from build123d import *

# Parameters (mm, degrees)
SKETCH1_W           = 121
SKETCH1_H           = 66
BOSS_EXTRUDE1_DEPTH = 3.8
SKETCH2_W           = 109
SKETCH2_H           = 58
CUT_EXTRUDE1_DEPTH  = 4.8
FILLET1_R           = 5
SKETCH3_W           = 20
SKETCH3_H           = 58
BOSS_EXTRUDE2_DEPTH = 3.8
FILLET2_R           = 3
SKETCH4_R           = 1
CUT_EXTRUDE2_DEPTH  = 4.8
BOSS_EXTRUDE3_DEPTH = 3.8
FILLET3_R           = 3
SKETCH6_W           = 3.8
SKETCH6_H           = 10
SKETCH6_W_2         = 10
SKETCH6_H_2         = 3.8
CUT_EXTRUDE3_DEPTH  = 4.8


with BuildPart() as part:
    # Sketch1 → Boss-Extrude1 (new body)
    with BuildSketch(Plane(origin=(0, 0, 0), x_dir=(1, 0, 0), z_dir=(0, 1, 0))):
        with Locations((60.5, -33)):
            Rectangle(SKETCH1_W, SKETCH1_H)
    extrude(amount=BOSS_EXTRUDE1_DEPTH)

    # Sketch2 → Cut-Extrude1 (cut, through all)
    with BuildSketch(Plane(origin=(0, 3.8, 0), x_dir=(1, 0, 0), z_dir=(0, 1, 0))):
        with Locations((60.5, -33)):
            Rectangle(SKETCH2_W, SKETCH2_H)
    extrude(amount=-CUT_EXTRUDE1_DEPTH, mode=Mode.SUBTRACT)

    # Fillet1
    fillet1_edges = [part.edges().sort_by_distance(p)[0] for p in [
        (115, 1.9, 4),
        (115, 1.9, 62),
        (6, 1.9, 62),
        (6, 1.9, 4),
    ]]
    fillet(fillet1_edges, radius=FILLET1_R)

    # Sketch3 → Boss-Extrude2 (add, through all)
    with BuildSketch(Plane(origin=(0, 3.8, 0), x_dir=(1, 0, 0), z_dir=(0, 1, 0))):
        with Locations((60.5, -33)):
            Rectangle(SKETCH3_W, SKETCH3_H)
    extrude(amount=-BOSS_EXTRUDE2_DEPTH)

    # Fillet2
    fillet2_edges = [part.edges().sort_by_distance(p)[0] for p in [
        (70.5, 1.9, 4),
        (70.5, 1.9, 62),
        (50.5, 1.9, 62),
        (50.5, 1.9, 4),
    ]]
    fillet(fillet2_edges, radius=FILLET2_R)

    # Sketch4 → Cut-Extrude2 (cut, through all)
    with BuildSketch(Plane(origin=(0, 3.8, 0), x_dir=(1, 0, 0), z_dir=(0, 1, 0))):
        with Locations((116.5, -61.5)):
            Circle(SKETCH4_R)
        with Locations((116.5, -4.5)):
            Circle(SKETCH4_R)
        with Locations((4.5, -4.5)):
            Circle(SKETCH4_R)
        with Locations((4.5, -61.5)):
            Circle(SKETCH4_R)
    extrude(amount=-CUT_EXTRUDE2_DEPTH, mode=Mode.SUBTRACT)

    # Sketch5 → Boss-Extrude3 (add, through all)
    with BuildSketch(Plane(origin=(0, 3.8, 0), x_dir=(1, 0, 0), z_dir=(0, 1, 0))):
        Polygon((0, 0), (-15, 0), (-15, -76), (136, -76), (136, 0), (121, 0), (121, -66), (0, -66), align=None)
    extrude(amount=-BOSS_EXTRUDE3_DEPTH)

    # Fillet3
    fillet3_edges = [part.edges().sort_by_distance(p)[0] for p in [
        (136, 1.9, 0),
        (136, 1.9, 76),
        (-15, 1.9, 76),
        (-15, 1.9, 0),
    ]]
    fillet(fillet3_edges, radius=FILLET3_R)

    # Sketch6 → Cut-Extrude3 (cut, through all)
    with BuildSketch(Plane.XZ):
        with Locations((131.1, 25)):
            Rectangle(SKETCH6_W, SKETCH6_H)
        with Locations((131.1, 45)):
            Rectangle(SKETCH6_W, SKETCH6_H)
        with Locations((131.1, 65)):
            Rectangle(SKETCH6_W, SKETCH6_H)
        with Locations((120.5, 71.1)):
            Rectangle(SKETCH6_W_2, SKETCH6_H_2)
        with Locations((100.5, 71.1)):
            Rectangle(SKETCH6_W_2, SKETCH6_H_2)
        with Locations((80.5, 71.1)):
            Rectangle(SKETCH6_W_2, SKETCH6_H_2)
        with Locations((60.5, 71.1)):
            Rectangle(SKETCH6_W_2, SKETCH6_H_2)
        with Locations((40.5, 71.1)):
            Rectangle(SKETCH6_W_2, SKETCH6_H_2)
        with Locations((20.5, 71.1)):
            Rectangle(SKETCH6_W_2, SKETCH6_H_2)
        with Locations((0.5, 71.1)):
            Rectangle(SKETCH6_W_2, SKETCH6_H_2)
        with Locations((-10.1, 65)):
            Rectangle(SKETCH6_W, SKETCH6_H)
        with Locations((-10.1, 45)):
            Rectangle(SKETCH6_W, SKETCH6_H)
        with Locations((-10.1, 25)):
            Rectangle(SKETCH6_W, SKETCH6_H)
    extrude(amount=-CUT_EXTRUDE3_DEPTH, mode=Mode.SUBTRACT)


solid = part.part
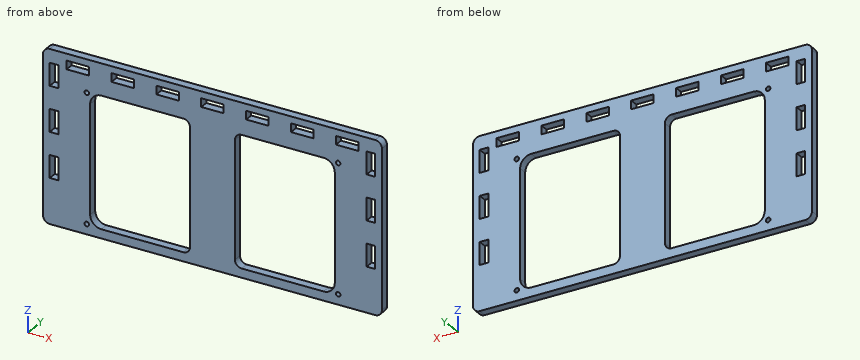
Verification items for the finished model (mm, model axes). Give positions to 0.01 mm unless a question says otherwise; leave off trailing zeros. Write each loop counter-clockwise with the first axis right and the second up, starting at its lowest first coordinate (ties: lowest second). Pieces come first, ordered by that corner, then holes. Notation, with made-up numbers: M 3,39 L 48,39 A13 ccw 48,47 Z; hole C 25.25,88.5 d1. An arc over 180 degrees is marked long. Put each result on its own line as item: value. Start each with the question number.
1. Section check B-B (x = 2). Record the cut outline in (y, z), and give its area (3 significant figures).
2. Section check A-A (z = 37). Record the cut outline in (x, y), and give its area (3 significant figures).
3. Scan lines: line 1 along X through (y, z) = (2.6, 21); line 2 along X through (y, z) = (0.9, 17); line 3 along Z through (x, y) = (102.5, 2.15). Record each from-to range of solid material in increasing order. Write a range as [from, to].
4. Section check D-D (y = 2.15). Give the number of separate pieces and of enclosed holes in the cut face, and give its area (3 significant figures).
5. Section check C-C (x = 23). Record the cut outline in (y, z).
Answer list:
1. outline: M 0,0 L 3.8,0 L 3.8,69.2 L 0,69.2 Z; M 0,73 L 3.8,73 L 3.8,76 L 0,76 Z
1. area: 274 mm2
2. outline: M -15,0 L 6,0 L 6,3.8 L -15,3.8 Z; M 50.5,0 L 70.5,0 L 70.5,3.8 L 50.5,3.8 Z; M 115,0 L 136,0 L 136,3.8 L 115,3.8 Z
2. area: 236 mm2
3. line 1: [-15, -12], [-8.2, 6], [50.5, 70.5], [115, 129.2], [133, 136]
3. line 2: [-15, 6], [50.5, 70.5], [115, 136]
3. line 3: [0, 4], [62, 69.2], [73, 76]
4. separate pieces: 1
4. enclosed holes: 19
4. area: 5,830 mm2
5. outline: M 0,0 L 3.8,0 L 3.8,4 L 0,4 Z; M 0,62 L 3.8,62 L 3.8,69.2 L 0,69.2 Z; M 0,73 L 3.8,73 L 3.8,76 L 0,76 Z
